For this review, take the finished solid that the model builds, in its own axes (mm). Face numbers are marked on the shaded views. A direction names the side the tool comes from. Round coordinates to 2 decimals unless told otherwise and drop trailing zeros. Loops run counter-clockwise (first coordinate to the right, second up) from the corner with the lowest first, then second, coordinate; pieces in that order, holes last.
1) Mouldability with a two-part tool opening along Z and no side actions: class the marked faces 1, 2 and 3 as pulls with the +Z half, pulls with the -Z half, needs draft (parallel to the pull), parting line crosses it, or undercut.
2) Take a section at D-D (y = 5.75). State the section outline as (x, z) points, then the cut area to 3 significant figures.
3) Tool access review of the marked faces 4 and 5: name each direction out of +Z, -Z, +X, -X, +Y, -Y from which nothing blocks a thin tool from reaching the whole face with its end or side.
4) Take a section at A-A (z = -2.7). State the section outline as (x, y) points.
5) Take a section at B-B (x = -27.75). State the section outline as (y, z) points, then the cut area to 3 significant figures.
6) Insertion check: pin 1 (1.6 mm diameter, centred on x = -4, y = 4, fed in from -Z); pin 2 (1.5 mm diameter, centred on x = -9, y = 5.5, fed in from +Z); pin 3 (2.5 mm diameter, centred on x = -4, z = -2.7, fed in from +Y); pin 4 (1.2 mm diameter, centred on x = -4, y = 3.7, fed in from -Z). Each pin has a flat end and moves straight along its axis. Give the tip position at first contact, or say it passes through.
7) Wall thickness on L1, parallel to Z at x = -26, y = 2.5; L2, parallel to Z at x = -4, y = 2.85; L3, parallel to X at y = 3, z = -8.5: over which ranges is each line inside the solid? List them lowest first.
8) Take a section at C-C (z = -12.5). State the section outline as (x, y) points, then the cut area to 3 significant figures.
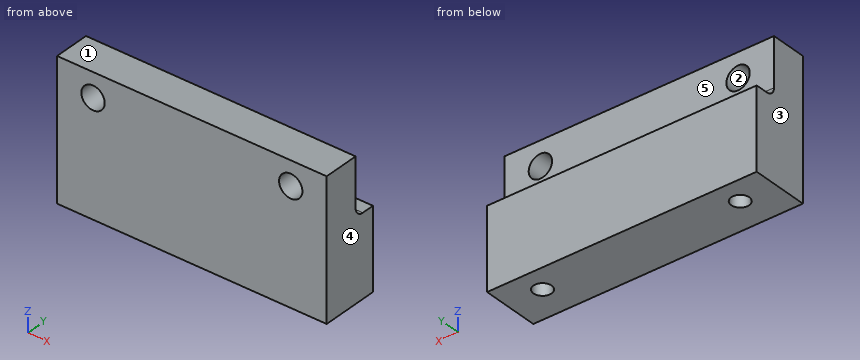
```python
from build123d import *

# Parameters (mm, degrees)
SKETCH1_W                 = 30
SKETCH1_H                 = 15.4
BOSS_EXTRUDE1_DEPTH       = 6.4
SKETCH4_R                 = 1.3
CUT_EXTRUDE3_DEPTH        = 7.4
SKETCH8_W                 = 11.4
SKETCH8_H                 = 2.4
CUT_EXTRUDE4_DEPTH        = 31
SKETCH9_R                 = 0.5
CUT_EXTRUDE5_DEPTH        = 7
M2X0_4_TAPPED_HOLE1_D     = 1.6
M2X0_4_TAPPED_HOLE1_DEPTH = 7
M2X0_4_TAPPED_HOLE1_TIP   = 0.480688495
SKETCH14_W                = 30
SKETCH14_H                = 5
BOSS_EXTRUDE2_DEPTH       = 2.4
SKETCH13_R                = 1
CUT_EXTRUDE6_DEPTH        = 7
FILLET1_R                 = 1


with BuildPart() as part:
    # Sketch1 → Boss-Extrude1 (new body)
    with BuildSketch(Plane(origin=(0, 0, 0), x_dir=(1, 0, 0), z_dir=(0, 1, 0))):
        with Locations((-15, 7.7)):
            Rectangle(SKETCH1_W, SKETCH1_H)
    extrude(amount=BOSS_EXTRUDE1_DEPTH)

    # Sketch4 → Cut-Extrude3 (cut, through all)
    with BuildSketch(Plane(origin=(0, 0, 0), x_dir=(1, 0, 0), z_dir=(0, 1, 0))):
        with Locations((-26, 2.7)):
            Circle(SKETCH4_R)
        with Locations((-4, 2.7)):
            Circle(SKETCH4_R)
    extrude(amount=CUT_EXTRUDE3_DEPTH, mode=Mode.SUBTRACT)

    # Sketch8 → Cut-Extrude4 (cut, through all)
    with BuildSketch(Plane(origin=(0, 0, 0), x_dir=(0, 0, -1), z_dir=(1, 0, 0))):
        with Locations((5.7, 5.2)):
            Rectangle(SKETCH8_W, SKETCH8_H)
    extrude(amount=-CUT_EXTRUDE4_DEPTH, mode=Mode.SUBTRACT)

    # Sketch9 → Cut-Extrude5 (cut)
    with BuildSketch(Plane(origin=(0, 0, -15.4), x_dir=(-1, 0, 0), z_dir=(0, 0, -1))):
        with Locations((4, 3.7)):
            Circle(SKETCH9_R)
        with Locations((26, 3.7)):
            Circle(SKETCH9_R)
    extrude(amount=-CUT_EXTRUDE5_DEPTH, mode=Mode.SUBTRACT)

    # M2x0.4 Tapped Hole1
    with Locations(Plane(origin=(0, 0, -15.4), x_dir=(-1, 0, 0), z_dir=(0, 0, -1))):
        with Locations((4, 3.7), (26, 3.7)):
            Hole(M2X0_4_TAPPED_HOLE1_D / 2, depth=M2X0_4_TAPPED_HOLE1_DEPTH)
            with Locations((0, 0, -(M2X0_4_TAPPED_HOLE1_DEPTH + M2X0_4_TAPPED_HOLE1_TIP / 2))):  # 118° drill point
                Cone(0, M2X0_4_TAPPED_HOLE1_D / 2, M2X0_4_TAPPED_HOLE1_TIP, mode=Mode.SUBTRACT)

    # Sketch14 → Boss-Extrude2 (add)
    with BuildSketch(Plane(origin=(0, 6.4, 0), x_dir=(1, 0, 0), z_dir=(0, 1, 0))):
        with Locations((-15, 8.9)):
            Rectangle(SKETCH14_W, SKETCH14_H)
    extrude(amount=-BOSS_EXTRUDE2_DEPTH)

    # Sketch13 → Cut-Extrude6 (cut)
    with BuildSketch(Plane(origin=(0, 0, -15.4), x_dir=(-1, 0, 0), z_dir=(0, 0, -1))):
        with Locations((4, 3.7)):
            Circle(SKETCH13_R)
        with Locations((26, 3.7)):
            Circle(SKETCH13_R)
    extrude(amount=-CUT_EXTRUDE6_DEPTH, mode=Mode.SUBTRACT)

    # Fillet1
    fillet1_edges = [part.edges().sort_by_distance(p)[0] for p in [
        (-15, 4, -6.4),
    ]]
    fillet(fillet1_edges, radius=FILLET1_R)


solid = part.part
```
Response:
1. face 1: pulls with the +Z half
1. face 2: undercut
1. face 3: needs draft
2. outline: (-30, -15.4) - (0, -15.4) - (0, -6.4) - (-30, -6.4) - close
2. area: 270 mm2
3. face 4: +Z, -Z, +X, +Y, -Y
3. face 5: +Z, +X, -X, +Y
4. outline: (-30, 0) - (-27.3, 0) - (-27.3, 4) - (-30, 4) - close; (-24.7, 0) - (-5.3, 0) - (-5.3, 4) - (-24.7, 4) - close; (-2.7, 0) - (0, 0) - (0, 4) - (-2.7, 4) - close
5. outline: (0, -15.4) - (6.4, -15.4) - (6.4, -6.4) - (5, -6.4) arc R1 cw to (4, -5.4) - (4, 0) - (0, 0) - close
5. area: 83.4 mm2
6. pin 1: stops at z = -15.4
6. pin 2: stops at z = -6.37
6. pin 3: passes through
6. pin 4: stops at z = -8.4
7. L1: z = -15.4 to -4, -1.4 to 0
7. L2: z = -8.4 to -4, -1.4 to 0
7. L3: x = -30 to -26.71, -25.29 to -4.71, -3.29 to 0
8. outline: (-30, 0) - (0, 0) - (0, 6.4) - (-30, 6.4) - close; hole circle Ø2 at (-26, 3.7); hole circle Ø2 at (-4, 3.7)
8. area: 186 mm2
